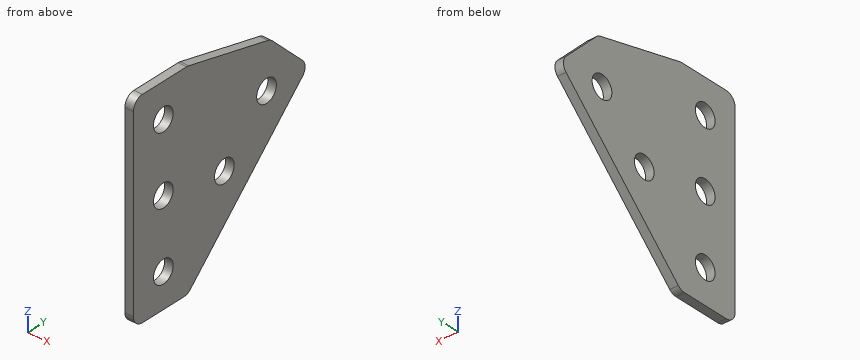
```python
from build123d import *

# Parameters (mm, degrees)
BOSS_EXTRUDE1_DEPTH = 2.5
SKETCH2_R           = 3.3
CUT_EXTRUDE1_DEPTH  = 3.5
LPATTERN1_COUNT     = 3
LPATTERN1_PITCH     = 20
SKETCH2_4_R         = 3.3
CUT_EXTRUDE2_DEPTH  = 3.5
LPATTERN2_COUNT     = 2
LPATTERN2_PITCH     = 20
FILLET1_R           = 3


with BuildPart() as part:
    # Sketch1 → Boss-Extrude1 (new body)
    with BuildSketch(Plane(origin=(0, 0, 0), x_dir=(0, 0, -1), z_dir=(1, 0, 0))):
        Polygon((-78.140120378, 0), (-18.140120378, 0), (-18.140120378, 18.140120378), (-58.68306962, 58.68306962), (-71.510071751, 45.856067489), (-78.140120378, 18.140120378), align=None)
    extrude(amount=BOSS_EXTRUDE1_DEPTH)

    # Sketch2 → Cut-Extrude1 (cut, through all)
    with BuildSketch(Plane(origin=(2.5, 0, 0), x_dir=(0, 0, -1), z_dir=(1, 0, 0))):
        with Locations((-28.140120378, 10)):
            Circle(SKETCH2_R)
    cut_extrude1 = extrude(amount=-CUT_EXTRUDE1_DEPTH, mode=Mode.SUBTRACT)

    # LPattern1: Cut-Extrude1 ×3
    with Locations(*[(0, 0, i * LPATTERN1_PITCH) for i in range(1, LPATTERN1_COUNT)]):
        add(cut_extrude1, mode=Mode.SUBTRACT)

    # Sketch2_4 → Cut-Extrude2 (cut, through all)
    with BuildSketch(Plane(origin=(2.5, 0, 0), x_dir=(0, 0, -1), z_dir=(1, 0, 0))):
        with Locations((-58.68306962, 44.540933996)):
            Circle(SKETCH2_4_R)
    cut_extrude2 = extrude(amount=-CUT_EXTRUDE2_DEPTH, mode=Mode.SUBTRACT)

    # LPattern2: Cut-Extrude2 ×2
    with Locations(*[Vector(0, -0.707106781, -0.707106781) * (i * LPATTERN2_PITCH) for i in range(1, LPATTERN2_COUNT)]):
        add(cut_extrude2, mode=Mode.SUBTRACT)

    # Fillet1
    fillet1_edges = [part.edges().sort_by_distance(p)[0] for p in [
        (1.25, 18.140120378, 78.140120378),
        (1.25, 45.856067489, 71.510071751),
        (1.25, 58.68306962, 58.68306962),
        (1.25, 18.140120378, 18.140120378),
        (1.25, 0, 18.140120378),
        (1.25, 0, 78.140120378),
    ]]
    fillet(fillet1_edges, radius=FILLET1_R)


solid = part.part
```
Part model, mm, in its own coordinate system. Coordinates: 2 decimals unless noted, no trailing zeros. Write each loop counter-clockwise with the first axis right and the second up, starting at its lowest first coordinate (ties: lowest second). Pieces come first, ordered by that corner, then holes.
Item 1: Slice it at D-D (x = 1.2). Write the cut outline in (y, z), and give its area (3 significant figures).
Item 2: Slice it at B-B (z = 50.5). Write the cut outline in (x, y).
Item 3: Slice it at A-A (y = 10). Write the cut outline in (x, z).
Item 4: Slice it at C-C (y = 29). Write the cut outline in (x, z), and give its area (3 significant figures).
Item 5: Pin check, flat tips, straight feed: pin 1 (4 mm diameter, centred on y = 44.54, z = 58.68, fed in from -X); pin 2 (10.5 mm diameter, centred on y = 10, z = 48.14, fed in from +X); pin 3 (1 mm diameter, centred on x = 1, y = 18.5, fed in from +Z). Stop position of each tip, or through.
Item 6: Probe line 1 (Z direction, x = 1.95, y = 10.5); line 2 (Z direction, x = 0.85, y = 47.5); line 3 (Y direction, x = 1.55, z = 45.5). List the from-to ranges inside material, lowest first.
Results found:
1. outline: (0, 21.14) arc R3 ccw to (3, 18.14) - (16.9, 18.14) arc R3 ccw to (19.02, 19.02) - (56.56, 56.56) arc R3 ccw to (56.56, 60.8) - (46.46, 70.91) arc R3 ccw to (45.03, 71.71) - (18.48, 78.06) arc R3 ccw to (17.79, 78.14) - (3, 78.14) arc R3 ccw to (0, 75.14) - close; hole circle Ø6.6 at (10, 28.14); hole circle Ø6.6 at (10, 48.14); hole circle Ø6.6 at (10, 68.14); hole circle Ø6.6 at (30.4, 44.54); hole circle Ø6.6 at (44.54, 58.68)
1. area: 2,260 mm2
2. outline: (0, 0) - (2.5, 0) - (2.5, 7.69) - (0, 7.69) - close; (0, 12.31) - (2.5, 12.31) - (2.5, 50.5) - (0, 50.5) - close
3. outline: (0, 18.14) - (2.5, 18.14) - (2.5, 24.84) - (0, 24.84) - close; (0, 31.44) - (2.5, 31.44) - (2.5, 44.84) - (0, 44.84) - close; (0, 51.44) - (2.5, 51.44) - (2.5, 64.84) - (0, 64.84) - close; (0, 71.44) - (2.5, 71.44) - (2.5, 78.14) - (0, 78.14) - close
4. outline: (0, 29) - (2.5, 29) - (2.5, 41.55) - (0, 41.55) - close; (0, 47.53) - (2.5, 47.53) - (2.5, 75.54) - (0, 75.54) - close
4. area: 101 mm2
5. pin 1: passes through
5. pin 2: stops at x = 2.5
5. pin 3: stops at z = 78.13
6. line 1: z = 18.14 to 24.88, 31.4 to 44.88, 51.4 to 64.88, 71.4 to 78.14
6. line 2: z = 47.5 to 57.22, 60.14 to 69.87
6. line 3: y = 0 to 8.02, 11.98 to 27.24, 33.56 to 45.5
